Input: dimensioned drawing with shaded views. Units: mm. Origin: part minimum x, y, z. A direction names the side the tool comes from. Give positions to 0.01 mm unless a question says otherwise; leave off trailing zeros. Write each loop counter-clockwise with the first axis right and the second up, starting at its lowest first coordinate (ties: lowest second). Pieces come first, ordered by that corner, then holes. Notation, with made-up numbers: (27, 32.25) -> (81, 32.25) arc R19 ccw to (81, 39.25) -> close; hole circle Ø8 at (-35, -24). An arc over 180 degrees is marked (long way). Answer as a JSON object with one key per item and string values.
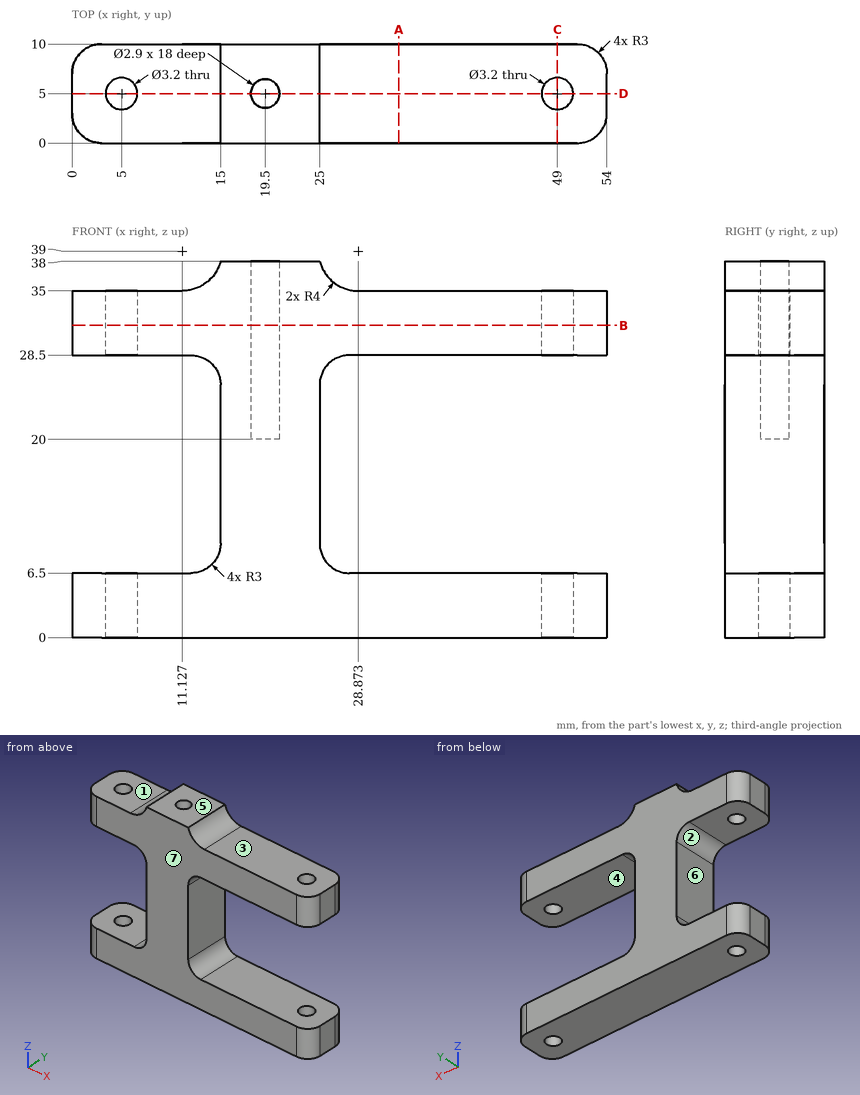
Q1. Set-up query: the marked faces 1, 2, 3 and 4. Return all of +Z, -Z, +X, -X, +Y, -Y with unobstructed straight access to the full face (end or side cutting, diameter ignored); none if empty.
Values:
{"face 1": "+Z, -X, +Y, -Y", "face 2": "-X, +Y, -Y", "face 3": "+Z, +X, +Y, -Y", "face 4": "+X, +Y, -Y"}
Q2. Cut plane B-B (z = 31.5). Return the cut outline in (x, y), and give its area (3 significant figures).
Values:
{"outline": "(0, 3) arc R3 ccw to (3, 0) -> (51, 0) arc R3 ccw to (54, 3) -> (54, 7) arc R3 ccw to (51, 10) -> (3, 10) arc R3 ccw to (0, 7) -> close; hole circle Ø3.2 at (5, 5); hole circle Ø2.9 at (19.5, 5); hole circle Ø3.2 at (49, 5)", "area": "510 mm²"}
Q3. Cut plane C-C (x = 49). Return the cut outline in (y, z), and give its area (3 significant figures).
Values:
{"outline": "(0, 0) -> (3.4, 0) -> (3.4, 6.5) -> (0, 6.5) -> close; (0, 28.5) -> (3.4, 28.5) -> (3.4, 35) -> (0, 35) -> close; (6.6, 0) -> (10, 0) -> (10, 6.5) -> (6.6, 6.5) -> close; (6.6, 28.5) -> (10, 28.5) -> (10, 35) -> (6.6, 35) -> close", "area": "88.4 mm²"}
Q4. Cut plane D-D (y = 5). State how many separate pieces and enclosed holes the cut face has, and give its area (3 significant figures).
Values:
{"separate pieces": "5", "enclosed holes": "0", "area": "830 mm²"}
Q5. Cut plane A-A (x = 33). Return the cut outline in (y, z), and give its area (3 significant figures).
Values:
{"outline": "(0, 0) -> (10, 0) -> (10, 6.5) -> (0, 6.5) -> close; (0, 28.5) -> (10, 28.5) -> (10, 35) -> (0, 35) -> close", "area": "130 mm²"}
Q6. First-contact query: P1, Ø5, axis at x = 3.5, y = 6.5, coming from the +Z side; P2, Ø1, axis at y = 9, z = 4, coming from the +X side; P3, Ø0.9, axis at x = 19.5, y = 5, coming from the +Z side. Flat tips, straight axial feed; report the tip coordinate or a pass-through.
Values:
{"P1": "z = 35", "P2": "x = 53.6", "P3": "z = 20"}
Q7. Material intervals for L1, parallel to Z at x = 34, y = 9; L2, parallel to X at y = 5, z = 24.75; L3, parallel to Y at x = 5, z = 31, sorted ascending. Write a range as from..to.
Values:
{"L1": "0..6.5, 28.5..35", "L2": "15..18.05, 20.95..25", "L3": "0..3.4, 6.6..10"}
Q8. Mould query, pull axis Z, two halves, no side actions, for the marked faces 5, 6 and 7. Classes: pulls with the +Z half, pulls with the -Z half, needs draft (parallel to the pull), parting line crosses it, or undercut.
Values:
{"face 5": "pulls with the +Z half", "face 6": "undercut", "face 7": "needs draft"}
